from build123d import *

# Parameters (mm, degrees)
FILLET1_R     = 0.396875
FILLET2_R     = 0.79375
CHAMFER1_SIZE = 0.254
CHAMFER2_SIZE = 0.127


with BuildPart() as part:
    # Sketch1 → Revolve1 (revolve)
    with BuildSketch(Plane.XY):
        Polygon((2.286, 0), (2.286, 12.7), (1.5875, 12.7), (1.5875, 44.45), (2.9845, 44.45), (2.9845, 3.175), (6.35, 3.175), (6.35, 0), align=None)
    revolve(axis=Axis((0, 5.299175628, 0), (0, -1, 0)))

    # Fillet1
    fillet1_edges = [part.edges().sort_by_distance(p)[0] for p in [
        (-2.286, 12.7, 0),
    ]]
    fillet(fillet1_edges, radius=FILLET1_R)

    # Fillet2
    fillet2_edges = [part.edges().sort_by_distance(p)[0] for p in [
        (-2.9845, 3.175, 0),
    ]]
    fillet(fillet2_edges, radius=FILLET2_R)

    # Chamfer1
    chamfer1_edges = [part.edges().sort_by_distance(p)[0] for p in [
        (-6.35, 0, 0),
        (-6.35, 3.175, 0),
        (-2.9845, 44.45, 0),
        (-1.5875, 44.45, 0),
        (-2.286, 0, 0),
    ]]
    chamfer(chamfer1_edges, length=CHAMFER1_SIZE)

    # Chamfer2
    chamfer2_edges = [part.edges().sort_by_distance(p)[0] for p in [
        (-1.5875, 12.7, 0),
    ]]
    chamfer(chamfer2_edges, length=CHAMFER2_SIZE)


solid = part.part
Work out the finished part from the listing and answer in its coordinate system (mm). A direction names the side the tool comes from. Round coordinates to 2 decimals unless told otherwise and drop trailing zeros. Write each loop counter-clockwise with the first axis right and the second up, starting at its lowest first coordinate (ties: lowest second). Pieces come first, ordered by that corner, then holes.
1) A cutting plane is placed at C-C (y = 5.5). Give the vertices of the cut face in (x, z).
2) Straight lines are drawn through the part: line 1 (Z direction, x = 0, y = 26.5); line 2 (Z direction, x = 0, y = 4.25); line 3 (Y direction, x = -3, z = 4) (3 decimals). For each, find the intervals that lie inside material, in ascending order.
3) Given pin 1 Ø6 at (x, y) = (4, 32.5) entering from +Z; pin 2 Ø6 at (x, y) = (0, 14) entering from -Z; pin 3 Ø2.5 at (x, z) = (0, 0) entering from +Y; pin 4 Ø1.9 at (x, z) = (0.5, -1) entering from -Y, each flat-ended and moving along its own axis, determine where each tip first touches the part or whether it passes through.
4) A cutting plane is placed at D-D (y = 41.5). Give the vertices of the cut face in (x, z) (1 decimal), plus the area to 3 significant figures.
5) A tool of negligible diameter and unlimited length cuts with its end or side. For faces 1 (the cylindrical face through (-0.647, 23.801, -2.914)), 2 (the cylindrical face through (-0.34, 28.73, -1.55)), from which of +Z, -Z, +X, -X, +Y, -Y can it reach the whole face along a straight path? Write none if from no direction.
6) The mould has two halves that part along X. Classify faces 3 (the cylindrical face through (-1.38, 1.57, -6.2)), 4 (the cylindrical face through (-0.5, 6.36, -2.23)), 5 (the flat face through (3, 0, 0)): pulls with the +X half, pulls with the -X half, needs draft (parallel to the pull), parting line crosses it, or undercut.
Completed:
1. outline: circle Ø5.97 at (0, 0); hole circle Ø4.57 at (0, 0)
2. line 1: z = -2.98 to -1.59, 1.59 to 2.98
2. line 2: z = -2.98 to -2.29, 2.29 to 2.98
2. line 3: y = 0 to 3.175
3. pin 1: stops at z = 2.81
3. pin 2: stops at z = -2.98
3. pin 3: passes through
3. pin 4: stops at y = 12.66
4. outline: circle Ø6 at (0, 0); hole circle Ø3.2 at (0, 0)
4. area: 20.1 mm2
5. face 1: +Y
5. face 2: +Y, -Y
6. face 3: parting line crosses it
6. face 4: undercut
6. face 5: needs draft
